```python
from build123d import *

# Parameters (mm, degrees)
SKETCH_1_R          = 1.5
EXTRUDE_1_DEPTH     = 18.5
SKETCH_2_R          = 1.5
EXTRUDE_2_DEPTH     = 3.5
SKETCH_3_R          = 2.6
SKETCH_3_R_2        = 1.5
EXTRUDE_3_DEPTH     = 0.5
EXTRUDE_START       = 4.5
SKETCH_7_R          = 1.5
EXTRUDE_4_DEPTH     = 4.5
CUT_EXTRUDE_START   = -1.5
SKETCH_4_R          = 1.5
SKETCH_4_R_2        = 1.25
CUT_EXTRUDE_1_DEPTH = 0.5
SKETCH_5_R          = 2
SKETCH_5_R_2        = 1
CUT_EXTRUDE_2_DEPTH = 2.5


with BuildPart() as part:
    # 草图1 → 凸台-拉伸1 (new body)
    with BuildSketch(Plane(origin=(0, 0, 0), x_dir=(0, 0, -1), z_dir=(1, 0, 0))):
        Circle(SKETCH_1_R)
    extrude(amount=EXTRUDE_1_DEPTH)

    # 草图2 → 凸台-拉伸2 (add)
    with BuildSketch(Plane.ZY.offset(-9)):
        with BuildLine():
            Line((-1.135781669, 2), (1.135781669, 2))
            ThreePointArc((1.135781669, 2), (0, -2.3), (-1.135781669, 2))
        make_face()
        Circle(SKETCH_2_R, mode=Mode.SUBTRACT)
    extrude(amount=-EXTRUDE_2_DEPTH)

    # 草图3 → 凸台-拉伸3 (add)
    with BuildSketch(Plane(origin=(12.5, 0, 0), x_dir=(0, 0, -1), z_dir=(1, 0, 0))):
        Circle(SKETCH_3_R)
        with Locations(Location((0, 0, 0), (0, 0, 180))):
            Circle(SKETCH_3_R_2, mode=Mode.SUBTRACT)
    extrude(amount=EXTRUDE_3_DEPTH)

    # 草图7 → 凸台-拉伸4 (add)
    with BuildSketch(Plane.ZY.offset(-9).offset(EXTRUDE_START)):
        with BuildLine():
            Line((-0.911921049, 1.78), (0.911921049, 1.78))
            ThreePointArc((0.911921049, 1.78), (0, -2), (-0.911921049, 1.78))
        make_face()
        with Locations(Location((0, 0, 0), (0, 0, 180))):
            Circle(SKETCH_7_R, mode=Mode.SUBTRACT)
    extrude(amount=-EXTRUDE_4_DEPTH)

    # 草图4 → 切除-拉伸1 (cut)
    with BuildSketch(Plane(origin=(18.5, 0, 0), x_dir=(0, 0, -1), z_dir=(1, 0, 0)).offset(CUT_EXTRUDE_START)):
        Circle(SKETCH_4_R)
        Circle(SKETCH_4_R_2, mode=Mode.SUBTRACT)
    extrude(amount=CUT_EXTRUDE_1_DEPTH, mode=Mode.SUBTRACT)

    # 草图5 → 切除-拉伸2 (cut)
    with BuildSketch(Plane.ZY):
        Circle(SKETCH_5_R)
        Circle(SKETCH_5_R_2, mode=Mode.SUBTRACT)
    extrude(amount=-CUT_EXTRUDE_2_DEPTH, mode=Mode.SUBTRACT)


solid = part.part
```
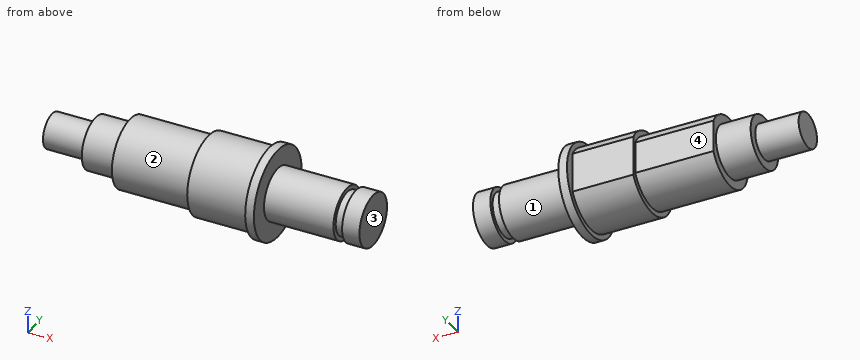
Can you work these out from the model? Positions are in its coordinate system, mm. Face numbers are marked on the shaded views. A direction names the side the tool comes from. Give positions to 0.01 mm unless a question says otherwise; leave off trailing zeros. Loops run counter-clockwise (first coordinate to the right, second up) from the corner with the lowest first, then second, coordinate; pieces in that order, holes last. Notation, with made-up numbers: M -11,-28.5 L 4,-28.5 A34 ccw 4,5.5 Z; hole C -19,44.5 d7. An arc over 180 degrees is marked long. Answer in a Markdown table with one row per item.
1. Suppose I cut it at C-C on x = 16. Write out the boundary of the cut face in (y, z), plus the area to 3 significant figures.
Taken from the geometry:
| item | result |
|---|---|
| outline | C 0,0 d3 |
| area | 7.07 mm² |
2. If I drill on line 1 along X through (y, z) = (0.3, -1.85); line 2 along Y through (x, z) = (10.25, -0.1); line 3 along X through (y, z) = (-1.7, -1.85), over which ranges is the centre line in solid material (lowest first)?
Taken from the geometry:
| item | result |
|---|---|
| line 1 | x = 4.5 to 13 |
| line 2 | y = -2.3 to 2 |
| line 3 | x = 12.5 to 13 |
3. Suppose I cut it at D-D on z = -1.7. Write out the boundary of the cut face in (x, y), plus the area to 3 significant figures.
Taken from the geometry:
| item | result |
|---|---|
| outline | M 4.5,-1.05 L 9,-1.05 L 9,-1.55 L 12.5,-1.55 L 12.5,-1.97 L 13,-1.97 L 13,1.97 L 12.5,1.97 L 12.5,1.55 L 9,1.55 L 9,1.05 L 4.5,1.05 Z |
| area | 22.3 mm² |
4. For pin 1 Ø1.5 at (x, z) = (7, 0) entering from +Y; pin 2 Ø1.5 at (x, y) = (2, 1.5) entering from -Z; pin 3 Ø2.5 at (x, z) = (11, 0) entering from +Y, each with a flat end and sliding along its axis, tell me the tip position at first contact or that it passes through.
Taken from the geometry:
| item | result |
|---|---|
| pin 1 | stops at y = 1.78 |
| pin 2 | stops at z = -1.17 |
| pin 3 | stops at y = 2 |
5. Which directions (+Z, -Z, +X, -X, +Y, -Y) give clear straight access to the entire face, cutting with the end or side of a thin tool? Please do the marked faces 1, 2, 3 and 4.
Taken from the geometry:
| item | result |
|---|---|
| face 1 | +X |
| face 2 | -X |
| face 3 | +Z, -Z, +X, +Y, -Y |
| face 4 | +Z, -Z, -X, +Y |
